Here's the drawing with two shaded views (mm, measured from the low corner). I have some questions. Give positions to 0.01 mm unless a question says otherwise; leave off trailing zeros. Write each loop counter-clockwise with the first axis right and the second up, starting at its lowest first coordinate (ties: lowest second). Pieces come first, ordered by that corner, then holes. Notation, with made-up numbers: (71.25, 43.5) - (113.25, 43.5) arc R20 ccw to (113.25, 57.5) - close; hole circle Ø4 at (59, -38.75). An arc over 180 degrees is marked (long way). Use one line per item in the form item = value. Start each with the question number.
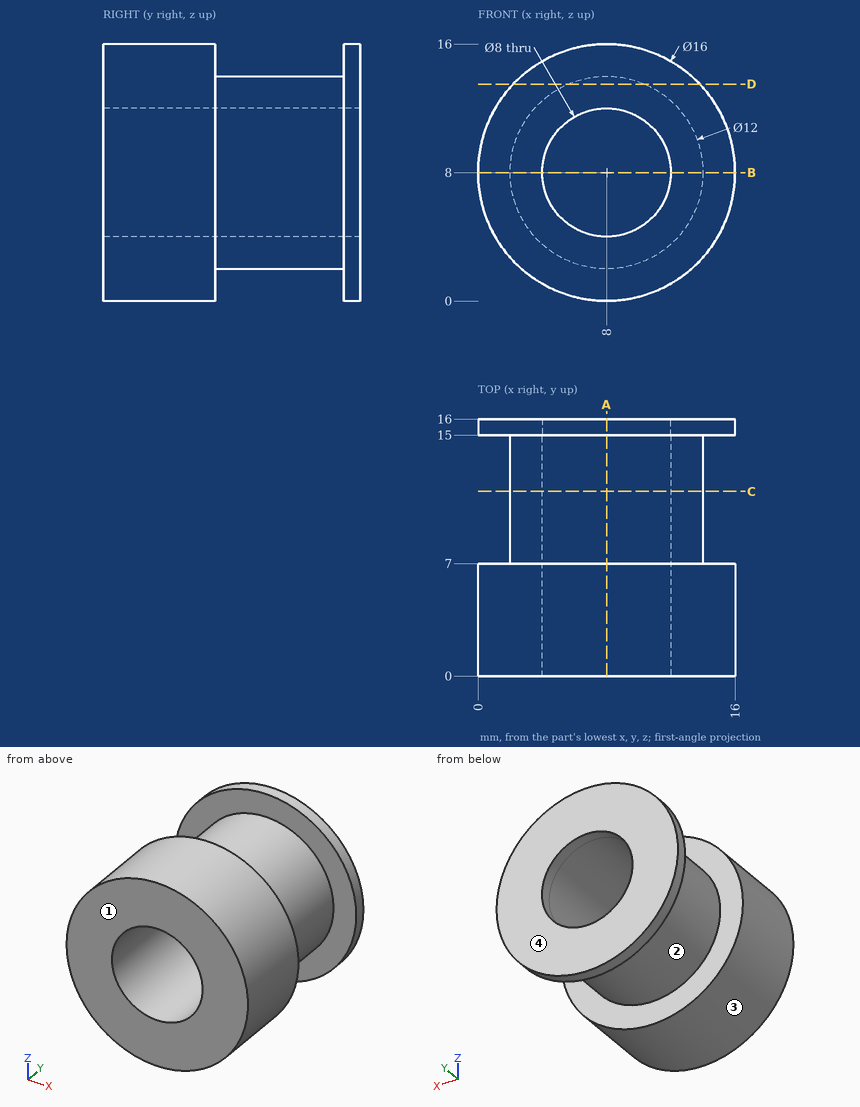
1. Please list where these lines run through material, in increasing order: line 1 (Y direction, x = 11.75, z = 13.5); line 2 (Z direction, x = 8, y = 5.25).
2. I want a section at C-C, the plane y = 11.5. List the corners of the cut face in (x, z) for me.
3. I want a section at D-D, the plane z = 13.5. List the corners of the cut face in (x, y) for me, then the cut area to 3 significant figures.
4. I want a section at A-A, the plane x = 8. List the corners of the cut face in (y, z) for me.
5. I want a section at B-B, the plane z = 8. List the corners of the cut face in (x, y) for me.
6. We'd pull the mould along Y, two halves only. Please class the marked faces 1, 2, 3 and 4: pulls with the +Y half, pulls with the -Y half, needs draft (parallel to the pull), parting line crosses it, or undercut.
7. For P1, Ø8, axis at y = 4.5, z = 12.5, coming from the +X side; P2, Ø5, axis at x = 8, z = 8, coming from the -Y side; P3, Ø5, axis at x = 2.5, y = 5.5, coming from the -Z side; P4, Ø2, axis at x = 6, y = 7, coming from the +Z side, each with a flat end and sliding along its axis, tell me the tip position at first contact or that it passes through.
Result sheet:
q1.line_1 = 0 to 7, 15 to 16
q1.line_2 = 0 to 4, 12 to 16
q2.outline = circle Ø12 at (8, 8); hole circle Ø8 at (8, 8)
q3.outline = (2.19, 0) - (13.81, 0) - (13.81, 7) - (10.4, 7) - (10.4, 15) - (13.81, 15) - (13.81, 16) - (2.19, 16) - (2.19, 15) - (5.6, 15) - (5.6, 7) - (2.19, 7) - close
q3.area = 131 mm2
q4.outline = (0, 0) - (7, 0) - (7, 2) - (15, 2) - (15, 0) - (16, 0) - (16, 4) - (0, 4) - close; (0, 12) - (16, 12) - (16, 16) - (15, 16) - (15, 14) - (7, 14) - (7, 16) - (0, 16) - close
q5.outline = (0, 0) - (4, 0) - (4, 16) - (0, 16) - (0, 15) - (2, 15) - (2, 7) - (0, 7) - close; (12, 0) - (16, 0) - (16, 7) - (14, 7) - (14, 15) - (16, 15) - (16, 16) - (12, 16) - close
q6.face_1 = pulls with the -Y half
q6.face_2 = undercut
q6.face_3 = needs draft
q6.face_4 = pulls with the +Y half
q7.P1 = 15.98
q7.P2 = through
q7.P3 = 0.58
q7.P4 = 15.94
